```python
from build123d import *

# Parameters (mm, degrees)
F0_R     = 1.6
F4_DEPTH = 3.5
F3_W     = 17
F3_H     = 14
F3_R     = 1.6
F7_DEPTH = 6
F8_R     = 1.6
F9_DEPTH = 2.6
F10_SIZE = 2


with BuildPart() as f4:
    # F0 (on Front) → F4 (new body, through all)
    with BuildSketch(Plane.XZ):
        with BuildLine():
            Line((-29.0554127395, 14.3491971341), (-44.0554127395, 14.3491971341))
            ThreePointArc((-44.0554127395, 14.3491971341), (-51.0554127395, 7.3491971341), (-44.0554127395, 0.3491971341))
            Line((-44.0554127395, 0.3491971341), (-29.0554127395, 0.3491971341))
            Line((-29.0554127395, 0.3491971341), (-29.0554127395, 14.3491971341))
        make_face()
        with Locations((-44.0554127395, 7.3491971341)):
            Circle(F0_R, mode=Mode.SUBTRACT)
    extrude(amount=-F4_DEPTH)


with BuildPart() as f6_1:
    # F6: instance of F4
    add(f4.part.mirror(Plane(origin=(0, 8.5, 0), x_dir=(-1, 0, 0), z_dir=(0, 1, 0))))


with BuildPart() as f4_1:
    add(f4.part)

    add(f6_1.part)  # F7 merges F6_1
    # F3 (on face) → F7 (join, through all)
    with BuildSketch(Plane.YZ.offset(-29.0554127395)):
        with Locations((8.5, 7.3491971341)):
            Rectangle(F3_W, F3_H)
        with Locations((8.5, 7.3491971341)):
            Circle(F3_R, mode=Mode.SUBTRACT)
    extrude(amount=-F7_DEPTH)

    # F8 (on face) → F9 (cut)
    with BuildSketch(Plane.XZ):
        Polygon((-42.3233619319, 10.3491971341), (-45.7874635471, 10.3491971341), (-47.5195143547, 7.3491971341), (-45.7874635471, 4.3491971341), (-42.3233619319, 4.3491971341), (-40.5913111244, 7.3491971341), align=None)
        with Locations((-44.0554127395, 7.3491971341)):
            Circle(F8_R, mode=Mode.SUBTRACT)
    extrude(amount=-F9_DEPTH, mode=Mode.SUBTRACT)

    # F10
    f10_edges = [f4_1.edges().sort_by_distance(p)[0] for p in [
        (-45.655413, 17, 7.349197),
        (-35.055413, 6.9, 7.349197),
    ]]
    chamfer(f10_edges, length=F10_SIZE)


solid = f4_1.part
```
CAD build for the part. Positions are in the model's coordinates, mm. A direction names the side the tool comes from. Round coordinates to 2 decimals unless told otherwise and drop trailing zeros. Loops run counter-clockwise (first coordinate to the right, second up) from the corner with the lowest first, then second, coordinate; pieces in that order, holes last. Notation, with made-up numbers: (-28.75, 72.25) - (3.25, 72.25) arc R34 ccw to (3.25, 108.25) - close; hole circle Ø6 at (-31, 28). An arc over 180 degrees is marked (long way). Return JSON: item names as keys, results as strings. Group by question number.
Q1. Flat gauge pins, fed straight in: pin 1 Ø7 at (x, z) = (-40, 9) entering from -Y; pin 2 Ø3.5 at (x, z) = (-44.06, 7.35) entering from +Y; pin 3 Ø1 at (y, z) = (9, 5) entering from -X; pin 4 Ø2.5 at (x, z) = (-44.06, 7.35) entering from +Y. Where does each tip first touch, or does it go through?
Q2. Band-saw the part on C-C on x = -49.25. Give the cut face in (y, z), plus the area to 3 significant figures.
Q3. Two-plate mould, pull along X, no slides. Class faces 4 (the face through (-42.577, 3.044, 6.736)), 5 (the face through (-51.054, 15.274, 7.503)), 6 (the face through (-38, 17, 7)): +X half, -X half, draft (parallel to the pull), parting line (faces both ways), or undercut.
Q4. Band-saw the part on A-A on y = 8.5. Give the cut face in (x, z).
Q5. Band-saw the part on B-B on y = 1.25. Give the cut face in (x, z).
Q6. Tool access for faces 1 (the face through (-41, 3.5, 7)), 2 (the face through (-31.027, 7.23, 6.376)), 3 (the face through (-46.64, 1.28, 8.87)): list every direction of +Z, -Z, +X, -X, +Y, -Y with a clear straight run to the whole face (end or side of a thin tool).
Q7. Band-saw the part on D-D on y = 3.75. Give the cut face in (x, z).
Q8. Drill centre lines: line 1 along Y through (x, z) = (-39, 3.5); line 2 along X through (y, z) = (12.75, 6.5); line 3 along Y through (x, z) = (-43.5, 4.5). Where is each one in solid material? Low to high. Write a range as [from, to].
Solutions:
{
 "1": {"pin 1": "stops at y = 0", "pin 2": "stops at y = 15.15", "pin 3": "stops at x = -34.36", "pin 4": "passes through"},
 "2": {"outline": "(0, 2.66) - (3.5, 2.66) - (3.5, 12.04) - (0, 12.04) - close; (13.5, 2.66) - (17, 2.66) - (17, 12.04) - (13.5, 12.04) - close", "area": "65.7 mm^2"},
 "3": {"face 4": "undercut", "face 5": "-X half", "face 6": "draft"},
 "4": {"outline": "(-35.06, 0.35) - (-29.06, 0.35) - (-29.06, 5.75) - (-33.06, 5.75) - (-35.06, 3.75) - close; (-35.06, 10.95) - (-33.06, 8.95) - (-29.06, 8.95) - (-29.06, 14.35) - (-35.06, 14.35) - close"},
 "5": {"outline": "(-44.06, 0.35) - (-29.06, 0.35) - (-29.06, 14.35) - (-44.06, 14.35) arc R7 ccw to start; hole (-47.52, 7.35) - (-45.79, 4.35) - (-42.32, 4.35) - (-40.59, 7.35) - (-42.32, 10.35) - (-45.79, 10.35) - close"},
 "6": {"face 1": "+Z, -Z, -X", "face 2": "+X, -X", "face 3": "-Y"},
 "7": {"outline": "(-35.06, 0.35) - (-29.06, 0.35) - (-29.06, 14.35) - (-35.06, 14.35) - close"},
 "8": {"line 1": "y = [0, 3.5], [13.5, 17]", "line 2": "x = [-35.06, -29.06]", "line 3": "y = [2.6, 3.5], [13.5, 16.3]"}
}
